from build123d import *

# Parameters (mm, degrees)
F0_R     = 175
F0_R_2   = 32.5
F0_R_3   = 10.5
F1_DEPTH = 20
F2_DEPTH = 25
F3_SIZE  = 2


with BuildPart() as f1:
    # F0 (on Top) → F1 (new body)
    with BuildSketch(Plane.XY):
        Circle(F0_R)
        Circle(F0_R_2, mode=Mode.SUBTRACT)
        Circle(F0_R_2)
        Circle(F0_R_3, mode=Mode.SUBTRACT)
    extrude(amount=-F1_DEPTH)

    # F0 (on Top) → F2 (join)
    with BuildSketch(Plane.XY):
        Circle(F0_R_2)
        Circle(F0_R_3, mode=Mode.SUBTRACT)
    extrude(amount=F2_DEPTH)

    # F3
    f3_edges = [f1.edges().sort_by_distance(p)[0] for p in [
        (-175, 0, 0),
        (-175, 0, -20),
        (-32.5, 0, 25),
    ]]
    chamfer(f3_edges, length=F3_SIZE)


solid = f1.part
Build history of the part. All positions in model axes, mm. A direction names the side the tool comes from. Give positions to 0.01 mm unless a question says otherwise; leave off trailing zeros. Order: outer loops, then holes, each group sorted by start corner. A loop starts at its lowest first (then second) coordinate and runs counter-clockwise, first axis right, second up. Notation, with made-up numbers: M -25.5,16 L 7.5,16 A32 ccw 7.5,44 Z; hole C 56,64 d7. An arc over 180 degrees is marked long. Use one line per item in the form item = value.
Q1. Slice it at A-A, the plane y = 0. Write the cut outline in (x, z), and give its area (3 significant figures).
Conclusion:
outline = M -175,-18 L -173,-20 L -10.5,-20 L -10.5,25 L -30.5,25 L -32.5,23 L -32.5,0 L -173,0 L -175,-2 Z; M 10.5,-20 L 173,-20 L 175,-18 L 175,-2 L 173,0 L 32.5,0 L 32.5,23 L 30.5,25 L 10.5,25 Z
area = 7,670 mm2
Q2. Wall check: probe 1 along Y at (x, z) = (0, 13.5); probe 2 along Z at (x, y) = (128.5, 37.5); probe 3 along Y at (x, z) = (0, -11). Give the ranges that are in metal, low to high.
Conclusion:
probe_1 = -32.5 to -10.5, 10.5 to 32.5
probe_2 = -20 to 0
probe_3 = -175 to -10.5, 10.5 to 175
Q3. Slice it at C-C, the plane z = -8. Write the cut outline in (x, y), and give its area (3 significant figures).
Conclusion:
outline = C 0,0 d350; hole C 0,0 d21
area = 95,900 mm2
Q4. Which spindle directions (+Z, -Z, +X, -X, +Y, -Y) get a long thin tool onto all of the face, cutting with end or side? Do faces 4 (the cylindrical face through (31, 9.76, 11.34)), 5 (the flat face through (-2, -36, -20)). Say none if no direction does.
Conclusion:
face_4 = +Z
face_5 = -Z, +X, -X, +Y, -Y
Q5. Pin check, flat tips, straight feed: P1, Ø4, axis at x = -91.5, z = 0.5, coming from the -Y side; P2, Ø5, axis at x = 118, z = -13, coming from the +Y side; P3, Ø8, axis at y = -1, z = 12.5, coming from the +X side; P4, Ø12.5, axis at x = 0, y = 0, coming from the -Z side. Stop position of each tip, or through.
Conclusion:
P1 = -148.89
P2 = 131.47
P3 = 32.5
P4 = through
Q6. Pull direction X, two halves, no side cores. Call faces 1 (the conical face through (165.131, 52.002, -19.875)), 2 (the flat face through (0, -13, 25)), 3 (the cylindrical face through (10, 3.2, 2.2)): released by +X, released by -X, zero draft, split by the parting line, or undercut.
Conclusion:
face_1 = split by the parting line
face_2 = zero draft
face_3 = undercut
Q7. Slice it at D-D, the plane z = 15.5. Write the cut outline in (x, y), and give its area (3 significant figures).
Conclusion:
outline = C 0,0 d65; hole C 0,0 d21
area = 2,970 mm2
